For this review, take the finished solid that the model builds, in its own axes (mm). Face numbers are marked on the shaded views. A direction names the side the tool comes from. Round coordinates to 2 decimals unless told otherwise and drop trailing zeros. Order: outer loops, then holes, each group sorted by start corner. A loop starts at its lowest first (then second) coordinate and runs counter-clockwise, first axis right, second up. Notation, with made-up numbers: M 34.5,-35 L 79.5,-35 A10 ccw 79.5,-31 Z; hole C -15,75 d9. An arc over 180 degrees is marked long. Answer in a Markdown table with one row per item. Add a question column.
```python
from build123d import *

# Parameters (mm, degrees)
F0_W     = 50
F0_H     = 30
F1_DEPTH = 15
F2_W     = 35.409173
F2_H     = 15.580036
F3_DEPTH = 10
F4_R     = 12.476899
F5_DEPTH = 25


with BuildPart() as f1:
    # F0 (on Top) → F1 (new body)
    with BuildSketch(Plane.XY):
        with Locations((-34.536691, 22.37889)):
            Rectangle(F0_W, F0_H)
    extrude(amount=F1_DEPTH)

    # F2 (on face) → F3 (join)
    with BuildSketch(Plane.XY.offset(15)):
        with Locations((-34.27608, 21.812051)):
            Rectangle(F2_W, F2_H)
    extrude(amount=F3_DEPTH)

    # F4 (on Top) → F5 (cut)
    with BuildSketch(Plane.XY):
        with Locations((-40.083185, 17.421314)):
            Circle(F4_R)
    extrude(amount=F5_DEPTH, mode=Mode.SUBTRACT)


solid = f1.part
```
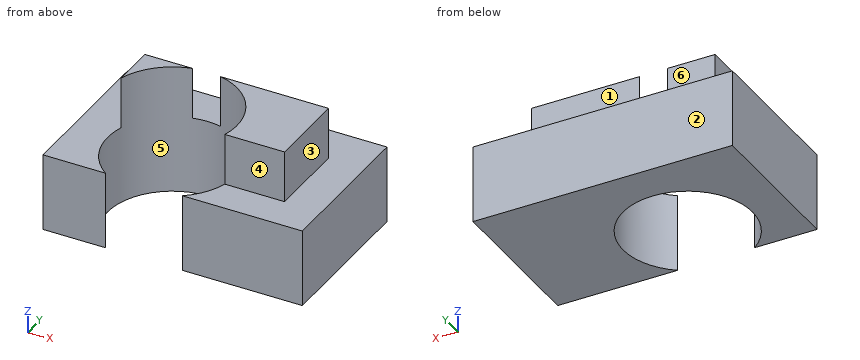
1. For the marked faces 1 and 2, list the 3-axis set-ups (+Z, -Z, +X, -X, +Y, -Y) from which the entire face can be reached by the end or side of a thin tool; tool diameter is ignored.
2. Consider section A-A on z = 21.5. Write out the cut boundary in (x, y).
3. Consider section C-C on y = 12.5. Write out the cut boundary in (x, z), plus the area to 3 significant figures.
4. The part is to be moulded in two halves that separate along Y. For the marked faces 3, 4, 5 and 6, say which applies: pulls with the +Y half, pulls with the -Y half, needs draft (parallel to the pull), parting line crosses it, or undercut.
5. Consider section D-D on x = -29.5. Write out the cut boundary in (y, z).
6. To check wall thickness, follow probe 1 along X at (y, z) = (17, 14.75); probe 2 along Z at (x, y) = (-14, 35.5); probe 3 along Y at (x, z) = (-18, 20). State the ranges of each line that lie inside material, in increasing order. Write a range as [from, to].
7. Clearance check with flat-ended pins moving along their axes: pin 1 Ø8 at (x, z) = (-23.5, 19.5) entering from +Y; pin 2 Ø5 at (y, z) = (24, 18.5) entering from +X; pin 3 Ø1 at (x, z) = (-17.5, 22) entering from -Y. State where each tip first meets the part, or that it passes through.
8. Consider section B-B on x = -19. Write out the cut boundary in (y, z), plus the area to 3 significant figures.
Solved:
| question | item | result |
|---|---|---|
| 1 | face 1 | +Z, +X, -X, +Y |
| 1 | face 2 | +Z, -Z, +X, -X, +Y |
| 2 | outline | M -51.98,21.18 A12.48 cw -42.79,29.6 L -51.98,29.6 Z; M -37.38,29.6 A12.48 cw -28.08,14.02 L -16.57,14.02 L -16.57,29.6 Z |
| 3 | outline | M -59.54,0 L -51.55,0 L -51.55,15 L -59.54,15 Z; M -28.62,0 L -9.54,0 L -9.54,15 L -28.62,15 Z |
| 3 | area | 406 mm^2 |
| 4 | face 3 | needs draft |
| 4 | face 4 | pulls with the -Y half |
| 4 | face 5 | undercut |
| 4 | face 6 | pulls with the +Y half |
| 5 | outline | M 7.38,0 L 10.81,0 L 10.81,15 L 7.38,15 Z; M 24.03,0 L 37.38,0 L 37.38,15 L 29.6,15 L 29.6,25 L 24.03,25 Z |
| 6 | probe 1 | x = [-59.54, -52.55], [-27.61, -9.54] |
| 6 | probe 2 | z = [0, 15] |
| 6 | probe 3 | y = [14.02, 29.6] |
| 7 | pin 1 | stops at y = 29.6 |
| 7 | pin 2 | stops at x = -16.57 |
| 7 | pin 3 | stops at y = 14.02 |
| 8 | outline | M 7.38,0 L 37.38,0 L 37.38,15 L 29.6,15 L 29.6,25 L 14.02,25 L 14.02,15 L 7.38,15 Z |
| 8 | area | 606 mm^2 |
